Autodesk Inventor part; units mm, degrees
ref_plane "YZ Plane" through (0, 0, 0) normal (1, 0, 0) x (0, 1, 0)
ref_plane "XZ Plane" through (0, 0, 0) normal (0, 1, 0) x (-1, 0, 0)
ref_plane "XY Plane" through (0, 0, 0) normal (0, 0, 1) x (1, 0, 0)
sketch "Szkic1" plane through (0, 0, 0) normal (1, 0, 0) x (0, 1, 0)
  line L0 (-37, 37) -> (37, 37)
  line L1 (37, 37) -> (37, -37)
  line L2 (37, -37) -> (-37, -37)
  line L3 (-37, -37) -> (-37, 37)
  line L4 (-37, 37) -> (37, -37) construction
  line L5 (37, 37) -> (-37, -37) construction
  point P0 (0, 0)
  dimension "d0" = 74
  dimension "d1" = 74
extrude "Wyciągnięcie proste1" add sketch "Szkic1" along normal blind 18
sketch "Szkic2" plane through (18, 0, 0) normal (1, 0, 0) x (0, 0, -1)
  circle A0 centre (-27.4, 31) radius 2.85
  line L0 (37, 37) -> (-37, 37)
  line L1 (-37, 37) -> (-37, -37)
  circle A1 centre (-27.4, 0) radius 2.85
  circle A2 centre (-27.4, -31) radius 2.85
  circle A3 centre (27.4, 31) radius 2.85
  line L2 (37, -37) -> (37, 37)
  circle A4 centre (27.4, 0) radius 2.85
  circle A5 centre (27.4, -31) radius 2.85
  line L3 (-29.8537, 35.25) -> (-24.9463, 35.25)
  line L4 (-24.9463, 35.25) -> (-22.4925, 31)
  line L5 (-22.4925, 31) -> (-24.9463, 26.75)
  line L6 (-24.9463, 26.75) -> (-29.8537, 26.75)
  line L7 (-29.8537, 26.75) -> (-32.3075, 31)
  line L8 (-32.3075, 31) -> (-29.8537, 35.25)
  line L9 (-29.8537, 4.25) -> (-24.9463, 4.25)
  line L10 (-24.9463, 4.25) -> (-22.4925, 0)
  line L11 (-22.4925, 0) -> (-24.9463, -4.25)
  line L12 (-24.9463, -4.25) -> (-29.8537, -4.25)
  line L13 (-29.8537, -4.25) -> (-32.3075, 0)
  line L14 (-32.3075, 0) -> (-29.8537, 4.25)
  line L15 (-29.8537, -26.75) -> (-24.9463, -26.75)
  line L16 (-24.9463, -26.75) -> (-22.4925, -31)
  line L17 (-22.4925, -31) -> (-24.9463, -35.25)
  line L18 (-24.9463, -35.25) -> (-29.8537, -35.25)
  line L19 (-29.8537, -35.25) -> (-32.3075, -31)
  line L20 (-32.3075, -31) -> (-29.8537, -26.75)
  line L21 (29.8537, 35.25) -> (32.3075, 31)
  line L22 (32.3075, 31) -> (29.8537, 26.75)
  line L23 (29.8537, 26.75) -> (24.9463, 26.75)
  line L24 (24.9463, 26.75) -> (22.4925, 31)
  line L25 (22.4925, 31) -> (24.9463, 35.25)
  line L26 (24.9463, 35.25) -> (29.8537, 35.25)
  line L27 (29.8537, 4.25) -> (32.3075, 0)
  line L28 (32.3075, 0) -> (29.8537, -4.25)
  line L29 (29.8537, -4.25) -> (24.9463, -4.25)
  line L30 (24.9463, -4.25) -> (22.4925, 0)
  line L31 (22.4925, 0) -> (24.9463, 4.25)
  line L32 (24.9463, 4.25) -> (29.8537, 4.25)
  line L33 (29.8537, -26.75) -> (32.3075, -31)
  line L34 (32.3075, -31) -> (29.8537, -35.25)
  line L35 (29.8537, -35.25) -> (24.9463, -35.25)
  line L36 (24.9463, -35.25) -> (22.4925, -31)
  line L37 (22.4925, -31) -> (24.9463, -26.75)
  line L38 (24.9463, -26.75) -> (29.8537, -26.75)
  point P0 (0, 0)
  point P1 (27.4, -26.75)
  dimension "d4" = 6
  dimension "d5" = 5.7
  dimension "d6" = 9.6
  dimension "d7" = 31
  dimension "d8" = 31
  dimension "d9" = 5.7
  dimension "d10" = 5.7
  dimension "d11" = 9.6
  dimension "d12" = 5.7
  dimension "d13" = 5.7
  dimension "d14" = 5.7
  dimension "d15" = 8.5
  dimension "d16" = 8.5
  dimension "d17" = 8.5
  dimension "d18" = 8.5
  dimension "d19" = 8.5
  dimension "d20" = 8.5
extrude "Wyciągnięcie proste2" cut sketch "Szkic2" against normal through all contours A0 | A1 | A2 | A3 | A4 | A5
extrude "Wyciągnięcie proste3" cut sketch "Szkic2" against normal blind 10 contours A0 | A1 | A2 | A3 | A4 | A5 | L3 L4 L5 L6 L7 L8 | L9 L10 L11 L12 L13 L14 | L15 L16 L17 L18 L19 L20 | L21 L22 L23 L24 L25 L26 | L27 L28 L29 L30 L31 L32 | L33 L34 L35 L36 L37 L38
sketch "Szkic3" plane through (0, -37, 37) normal (0, 0, 1) x (1, 0, 0)
  line L0 (0, 0) -> (0, 74)
  line L1 (0, 72.5) -> (2, 72.5)
  line L2 (2, 72.5) -> (2, 63.5)
  line L3 (2, 63.5) -> (0, 63.5)
  line L4 (0, 63.5) -> (0, 72.5)
  line L5 (0, 74) -> (18, 74)
  line L6 (0, 10.5) -> (2, 10.5)
  line L7 (2, 10.5) -> (2, 1.5)
  line L8 (2, 1.5) -> (0, 1.5)
  line L9 (0, 1.5) -> (0, 10.5)
  point P0 (0, 37)
  point P1 (0, 1.5)
  point P2 (0, 63.5)
  dimension "d25" = 1.5
  dimension "d26" = 9
  dimension "d27" = 2
  dimension "d28" = 2
  dimension "d29" = 9
  dimension "d30" = 1.5
extrude "Wyciągnięcie proste4" cut sketch "Szkic3" against normal through all
properties part number "Y_end_cover" material "Tworzywo sztuczne ABS"
Read the model definition and answer for the solid it produces. Units are mm, in the model's axes. A direction names the side the tool comes from. Coordinates: 2 decimals unless noted, no trailing zeros. Loops run counter-clockwise (first coordinate to the right, second up) from the corner with the lowest first, then second, coordinate; pieces in that order, holes last. Notation, with made-up numbers: (4, 29.25) -> (54, 29.25) arc R17 ccw to (54, 39.25) -> close; hole circle Ø8 at (-19.75, 80). An arc over 180 degrees is marked (long way). Write item = value, one per line. Start each with the question number.
1) The mould has two halves that part along Y. Classify faces 4 (the face through (9, 1, -37)), 5 (the face through (13.07, 2.095, -23.702)): pulls with the +Y half, pulls with the -Y half, needs draft (parallel to the pull), parting line crosses it, or undercut.
2) The part is cut by section B-B, the plane z = -27.4. State how many separate pieces and enclosed holes the cut face has, plus the area to 3 significant figures.
3) Find the intervals of material crossed by L1, parallel to Y at x = 4.5, z = 27.4; L2, parallel to Z at x = 6.75, y = -28.5; L3, parallel to Y at x = 1.5, z = 15.5, in increasing order. Write a range as from..to.
4) The part is cut by section A-A, the plane x = 7. Determine the outline of the cut face in (y, z), plus the area to 3 significant figures.
5) Given P1, Ø5, axis at y = 31, z = 27.4, coming from the +X side; P2, Ø7.5, axis at y = -31, z = -27.4, coming from the +X side, each flat-ended and moving along its own axis, determine where each tip first touches the part or whether it passes through.
6) The part is cut by section C-C, the plane y = 2. Determine the outline of the cut face in (x, z).
7) The part is cut by section D-D, the plane z = -4.5. Determine the outline of the cut face in (x, y).
8) For faces 1 (the face through (8, 33, 25)), 2 (the face through (4.056, 0.125, 30.247)), 3 (the face through (2, 31, 1)), determine the directions among +Z, -Z, +X, -X, +Y, -Y from which every point of the face is accessible in a straight line to the end or side of a thin tool.
Result:
q1.face_4 = needs draft
q1.face_5 = undercut
q2.separate_pieces = 4
q2.enclosed_holes = 0
q2.area = 927 mm²
q3.L1 = -37..-33.85, -28.15..-2.85, 2.85..28.15, 33.85..37
q3.L2 = -37..-28.77, -26.03..26.03, 28.77..37
q3.L3 = -37..-35.5, -26.5..26.5, 35.5..37
q4.outline = (-37, -37) -> (37, -37) -> (37, 37) -> (-37, 37) -> close; hole circle Ø5.7 at (-31, -27.4); hole circle Ø5.7 at (-31, 27.4); hole circle Ø5.7 at (0, -27.4); hole circle Ø5.7 at (0, 27.4); hole circle Ø5.7 at (31, -27.4); hole circle Ø5.7 at (31, 27.4)
q4.area = 5,320 mm²
q5.P1 = through
q5.P2 = 8
q6.outline = (0, -37) -> (18, -37) -> (18, -31.15) -> (8, -31.15) -> (8, -29.43) -> (0, -29.43) -> close; (0, -25.37) -> (8, -25.37) -> (8, -23.65) -> (18, -23.65) -> (18, 23.65) -> (8, 23.65) -> (8, 25.37) -> (0, 25.37) -> close; (0, 29.43) -> (8, 29.43) -> (8, 31.15) -> (18, 31.15) -> (18, 37) -> (0, 37) -> close
q7.outline = (0, -37) -> (18, -37) -> (18, 37) -> (0, 37) -> (0, 35.5) -> (2, 35.5) -> (2, 26.5) -> (0, 26.5) -> (0, -26.5) -> (2, -26.5) -> (2, -35.5) -> (0, -35.5) -> close
q8.face_1 = +X
q8.face_2 = +X, -X
q8.face_3 = +Z, -Z, -X
